```python
from build123d import *

# Parameters (mm, degrees)
F0_W     = 40
F0_H     = 35
F0_R     = 9.525
F1_DEPTH = 8
F2_R     = 4.1
F3_DEPTH = 4
F4_R     = 4.1
F5_DEPTH = 4
F6_R     = 1.55
F7_DEPTH = 8
F6_R_2   = 2.85
F8_DEPTH = 5


with BuildPart() as f1:
    # F0 (on Top) → F1 (new body)
    with BuildSketch(Plane.XY):
        Rectangle(F0_W, F0_H)
        Circle(F0_R, mode=Mode.SUBTRACT)
    extrude(amount=F1_DEPTH)

    # F2 (on face) → F3 (join)
    with BuildSketch(Plane(origin=(-20, 0, 0), x_dir=(0, -1, 0), z_dir=(-1, 0, 0))):
        with BuildLine():
            Line((-17.5, 0), (-7.445494, -25.579978))
            ThreePointArc((-7.445494, -25.579978), (0, -30.65344), (7.445494, -25.579978))
            Line((7.445494, -25.579978), (17.5, 0))
            Line((17.5, 0), (-17.5, 0))
        make_face()
        with Locations((0, -22.65344)):
            Circle(F2_R, mode=Mode.SUBTRACT)
    extrude(amount=-F3_DEPTH)

    # F4 (on face) → F5 (join)
    with BuildSketch(Plane.YZ.offset(20)):
        with BuildLine():
            Line((17.5, 0), (-17.5, 0))
            Line((-17.5, 0), (-7.445494, -25.579978))
            ThreePointArc((-7.445494, -25.579978), (0, -30.65344), (7.445494, -25.579978))
            Line((7.445494, -25.579978), (17.5, 0))
        make_face()
        with Locations((0, -22.65344)):
            Circle(F4_R, mode=Mode.SUBTRACT)
    extrude(amount=-F5_DEPTH)

    # F6 (on face) → F7 (cut, through all)
    with BuildSketch(Plane.XY.offset(8)):
        with Locations((-10, 10)):
            Circle(F6_R)
        with Locations((10, 10)):
            Circle(F6_R)
        with Locations((-10, -10)):
            Circle(F6_R)
        with Locations((10, -10)):
            Circle(F6_R)
    extrude(amount=-F7_DEPTH, mode=Mode.SUBTRACT)

    # F6 (on face) → F8 (cut)
    with BuildSketch(Plane.XY.offset(8)):
        with Locations((-10, 10)):
            Circle(F6_R_2)
        with Locations((-10, 10)):
            Circle(F6_R, mode=Mode.SUBTRACT)
        with Locations((-10, -10)):
            Circle(F6_R_2)
        with Locations((-10, -10)):
            Circle(F6_R, mode=Mode.SUBTRACT)
        with Locations((10, 10)):
            Circle(F6_R_2)
        with Locations((10, 10)):
            Circle(F6_R, mode=Mode.SUBTRACT)
        with Locations((10, -10)):
            Circle(F6_R_2)
        with Locations((10, -10)):
            Circle(F6_R, mode=Mode.SUBTRACT)
    extrude(amount=-F8_DEPTH, mode=Mode.SUBTRACT)


solid = f1.part
```
Here's how the part is built. I have some questions about the finished solid (model axes, mm). A direction names the side the tool comes from. Coordinates: 2 decimals unless noted, no trailing zeros. Order: outer loops, then holes, each group sorted by start corner. A loop starts at its lowest first (then second) coordinate and runs counter-clockwise, first axis right, second up.
1) Imagine slicing it at B-B on x = 0. List the corners of the cut face in (y, z) for me (3 decimals), and give its area (3 significant figures).
2) Will these pins go through, and if not, where does the flat tip stop? pin 1 (1 mm diameter, centred on x = 8.5, y = 0.5, fed in from -Z); pin 2 (4 mm diameter, centred on x = -10, y = 10, fed in from -Z); pin 3 (8 mm diameter, centred on x = 13, z = -12, fed in from +Y); pin 4 (5 mm diameter, centred on x = -10, y = -10, fed in from +Z).
3) We'd pull the mould along Z, two halves only. Please class faces 4 (the face through (18.03, 12.4, -12.97)), 5 (the face through (18.03, 1.89, -26.29)), 6 (the face through (-11.23, -10.94, 1.52)): +Z half, -Z half, draft (parallel to the pull), parting line (faces both ways), or undercut.
4) Imagine slicing it at A-A on y = 0. List the corners of the cut face in (x, z) for me (3 decimals), and give its area (3 significant figures).
5) Imagine slicing it at D-D on y = -11. List the corners of the cut face in (x, z) for me.
6) I need wall thicknesses on line 1 (Y direction, x = 10, z = 1.45); line 2 (X direction, y = 4, z = -20); line 3 (Y direction, x = -10, z = 5.15). Which ranges of each line are inside material? Lowest first, please.
7) Imagine slicing it at C-C on z = -13.5. List the corners of the cut face in (x, y) for me, and give its area (3 significant figures).
8) Which directions (+Z, -Z, +X, -X, +Y, -Y) give clear straight access to the entire face, cutting with the end or side of a thin tool? Please do faces 1 (the face through (-7.559, -5.796, 3.944)), 2 (the face through (16, 0, -12)), 3 (the face through (-12.847, -9.875, 5.535)).
Response values:
1. outline: (-17.5, 0) - (-9.525, 0) - (-9.525, 8) - (-17.5, 8) - close; (9.525, 0) - (17.5, 0) - (17.5, 8) - (9.525, 8) - close
1. area: 128 mm2
2. pin 1: passes through
2. pin 2: stops at z = 0
2. pin 3: stops at y = 13.82
2. pin 4: stops at z = 3
3. face 4: -Z half
3. face 5: undercut
3. face 6: draft
4. outline: (-20, -30.653) - (-16, -30.653) - (-16, -26.753) - (-20, -26.753) - close; (-20, -18.553) - (-16, -18.553) - (-16, 0) - (-9.525, 0) - (-9.525, 8) - (-20, 8) - close; (9.525, 0) - (16, 0) - (16, -18.553) - (20, -18.553) - (20, 8) - (9.525, 8) - close; (16, -30.653) - (20, -30.653) - (20, -26.753) - (16, -26.753) - close
4. area: 347 mm2
5. outline: (-20, -16.54) - (-16, -16.54) - (-16, 0) - (-11.18, 0) - (-11.18, 3) - (-12.67, 3) - (-12.67, 8) - (-20, 8) - close; (-8.82, 0) - (8.82, 0) - (8.82, 3) - (7.33, 3) - (7.33, 8) - (-7.33, 8) - (-7.33, 3) - (-8.82, 3) - close; (11.18, 0) - (16, 0) - (16, -16.54) - (20, -16.54) - (20, 8) - (12.67, 8) - (12.67, 3) - (11.18, 3) - close
6. line 1: y = -17.5 to -11.55, -8.45 to 8.45, 11.55 to 17.5
6. line 2: x = -20 to -16, 16 to 20
6. line 3: y = -17.5 to -12.85, -7.15 to 7.15, 12.85 to 17.5
7. outline: (-20, -12.19) - (-16, -12.19) - (-16, 12.19) - (-20, 12.19) - close; (16, -12.19) - (20, -12.19) - (20, 12.19) - (16, 12.19) - close
7. area: 195 mm2
8. face 1: +Z, -Z
8. face 2: -Z, +Y, -Y
8. face 3: +Z
